Build history of the part. All positions in model axes, mm. A direction names the side the tool comes from. Give positions to 0.01 mm unless a question says otherwise; leave off trailing zeros. Order: outer loops, then holes, each group sorted by start corner. A loop starts at its lowest first (then second) coordinate and runs counter-clockwise, first axis right, second up. Notation, with made-up numbers: (28.25, -21.75) -> (50.25, -21.75) arc R18 ccw to (50.25, 10.25) -> close; hole circle Ø10 at (1, 69.5). An arc over 180 degrees is marked (long way). Use a Markdown table: item, result. Add a question column.
```python
from build123d import *

# Parameters (mm, degrees)
SKETCH1_R                             = 45
BOSS_EXTRUDE1_DEPTH                   = 8
TAP_DRILL_FOR_M2X0_4_TAP1_D           = 1.6
TAP_DRILL_FOR_M2X0_4_TAP1_CSINK_D     = 1.65
TAP_DRILL_FOR_M2X0_4_TAP1_CSINK_ANGLE = 90
SKETCH7_W                             = 6
SKETCH7_H                             = 23.5
CUT_EXTRUDE1_DEPTH                    = 4.1
FILLET1_R                             = 2
BOSS_EXTRUDE2_DEPTH                   = 6
M2_CLEARANCE_HOLE3_D                  = 2.4
SKETCH17_R                            = 1.75
CUT_EXTRUDE2_DEPTH                    = 67.666933473
FILLET1_OF_MIRROR1_R                  = 2


with BuildPart() as part:
    # Sketch1 → Boss-Extrude1 (new body)
    with BuildSketch(Plane(origin=(0, 0, 0), x_dir=(1, 0, 0), z_dir=(0, 1, 0))):
        with Locations(Location((0, 0, 0), (0, 0, 270))):
            Circle(SKETCH1_R)
        Polygon((-15, -36.25), (-15, -4.25), (-20, -4.25), (-20, -5.75), (-26, -5.75), (-26, -4.25), (-34, -4.25), (-34, -11), (-42, -11), (-42, 11), (-34, 11), (-34, 4.25), (-26, 4.25), (-26, 5.75), (-20, 5.75), (-20, 4.25), (-15, 4.25), (-15, 36.25), (15, 36.25), (15, 4.25), (20, 4.25), (20, 5.75), (26, 5.75), (26, 4.25), (34, 4.25), (34, 11), (42, 11), (42, -11), (34, -11), (34, -4.25), (26, -4.25), (26, -5.75), (20, -5.75), (20, -4.25), (15, -4.25), (15, -36.25), align=None, mode=Mode.SUBTRACT)
    extrude(amount=BOSS_EXTRUDE1_DEPTH)

    # Sketch3 → Revolve1 (revolve)
    with BuildSketch(Plane.XY, mode=Mode.PRIVATE) as revolve1_sk:
        with BuildLine():
            Line((-45, 5.8), (-45, 2.2))
            ThreePointArc((-45, 2.2), (-46.8, 4), (-45, 5.8))
        make_face()
    revolve(revolve1_sk.sketch.rotate(Axis((0, 8.4, 0), (0, -1, 0)), 270), axis=Axis((0, 8.4, 0), (0, -1, 0)))

    # Tap Drill for M2x0.4 Tap1 (through all)
    with Locations(Plane(origin=(0, 8, 0), x_dir=(1, 0, 0), z_dir=(0, 1, 0))):
        with Locations((-19.480791822, 19.480791822), (19.480791822, 19.480791822), (19.480791822, -19.480791822), (-19.480791822, -19.480791822)):
            CounterSinkHole(TAP_DRILL_FOR_M2X0_4_TAP1_D / 2, TAP_DRILL_FOR_M2X0_4_TAP1_CSINK_D / 2, counter_sink_angle=TAP_DRILL_FOR_M2X0_4_TAP1_CSINK_ANGLE)

    # Sketch7 → Cut-Extrude1 (cut)
    with BuildSketch(Plane(origin=(0, 8, 0), x_dir=(1, 0, 0), z_dir=(0, 1, 0))):
        with Locations((-23, 0)):
            Rectangle(SKETCH7_W, SKETCH7_H)
    cut_extrude1 = extrude(amount=-CUT_EXTRUDE1_DEPTH, mode=Mode.SUBTRACT)

    # Fillet1
    fillet1_edges = [part.edges().sort_by_distance(p)[0] for p in [
        (-20, 5.95, -11.75),
        (-26, 5.95, 11.75),
        (-26, 5.95, -11.75),
        (-20, 5.95, 11.75),
    ]]
    fillet(fillet1_edges, radius=FILLET1_R)

    # Sketch8 → Boss-Extrude2 (add)
    with BuildSketch(Plane.ZY.offset(20)):
        with BuildLine():
            Line((-5.499090834, 3.9), (-10.499090834, 3.9))
            ThreePointArc((-10.499090834, 3.9), (0, -6.499567055), (10.499090834, 3.9))
            Line((10.499090834, 3.9), (5.499090834, 3.9))
            ThreePointArc((5.499090834, 3.9), (0, -1.5), (-5.499090834, 3.9))
        make_face()
    boss_extrude2 = extrude(amount=BOSS_EXTRUDE2_DEPTH)

    # M2 Clearance Hole3 (through all)
    with Locations(Plane(origin=(0, 3.9, 0), x_dir=(1, 0, 0), z_dir=(0, 1, 0))):
        with Locations((-23, 8.624545417), (-23, -8.624545417)):
            m2_clearance_hole3 = Hole(M2_CLEARANCE_HOLE3_D / 2)

    # Sketch17 → Cut-Extrude2 (cut, through all)
    with BuildSketch(Plane.XZ):
        with Locations((-23, -8.624545417)):
            Circle(SKETCH17_R)
        with Locations((-23, 8.624545417)):
            Circle(SKETCH17_R)
    cut_extrude2 = extrude(amount=CUT_EXTRUDE2_DEPTH, mode=Mode.SUBTRACT)

    # Mirror1: Cut-Extrude1, Boss-Extrude2, M2 Clearance Hole3, Cut-Extrude2 across plane
    add(cut_extrude1.mirror(Plane(origin=(0, 0, 0), x_dir=(0, 0, 1), z_dir=(1, 0, 0))), mode=Mode.SUBTRACT)
    add(boss_extrude2.mirror(Plane(origin=(0, 0, 0), x_dir=(0, 0, 1), z_dir=(1, 0, 0))))
    add(m2_clearance_hole3.mirror(Plane(origin=(0, 0, 0), x_dir=(0, 0, 1), z_dir=(1, 0, 0))), mode=Mode.SUBTRACT)
    add(cut_extrude2.mirror(Plane(origin=(0, 0, 0), x_dir=(0, 0, 1), z_dir=(1, 0, 0))), mode=Mode.SUBTRACT)

    # Fillet1 of Mirror1
    fillet1_of_mirror1_edges = [part.edges().sort_by_distance(p)[0] for p in [
        (20, 5.95, -11.75),
        (26, 5.95, 11.75),
        (26, 5.95, -11.75),
        (20, 5.95, 11.75),
    ]]
    fillet(fillet1_of_mirror1_edges, radius=FILLET1_OF_MIRROR1_R)


solid = part.part
```
(1) Mould opens along Z. For faces 1 (the face through (-30, 4, -4.25)), 2 (the face through (-19, 8, 9)), 3 (the face through (-17.235, 6.885, 41.569)) say: released by +Z, released by -Z, zero draft, split by the parting line, or undercut.
(2) Wall check: probe 1 along X at (y, z) = (7, -0.5); probe 2 along X at (y, z) = (4.25, -9); probe 3 along X at (y, z) = (-4.25, 6). Give the ranges that are in metal, low to high.
(3) Pin check, flat tips, straight feed: pin 1 Ø7.5 at (y, z) = (-3, 3.5) entering from +X; pin 2 Ø6 at (y, z) = (5, 7) entering from +X; pin 3 Ø2 at (x, z) = (-23, 8.62) entering from -Y; pin 4 Ø1.7 at (y, z) = (6, -7) entering from +X. Stop position of each tip, or through.
(4) Band-saw the part on B-B on z = 0. Give the cut face in (x, y), plus the area to 3 significant figures.
(5) Band-saw the part on A-A on x = 0. Give the cut face in (y, z).
(6) Tool access for faces 4 (the face through (23, 6, -11.75)), 5 (the face through (-17.235, 1.085, 41.569)), 6 (the face through (42, 4, 0)): list every direction of +Z, -Z, +X, -X, +Y, -Y with a clear straight run to the whole face (end or side of a thin tool).
Response:
| question | item | result |
|---|---|---|
| 1 | face 1 | undercut |
| 1 | face 2 | zero draft |
| 1 | face 3 | split by the parting line |
| 2 | probe 1 | x = -45 to -42, 42 to 45 |
| 2 | probe 2 | x = -45.91 to -42, -34 to -26, -20 to -15, 15 to 20, 26 to 34, 42 to 45.91 |
| 2 | probe 3 | x = -26 to -20, 20 to 26 |
| 3 | pin 1 | stops at x = 44.98 |
| 3 | pin 2 | stops at x = 46.61 |
| 3 | pin 3 | passes through |
| 3 | pin 4 | stops at x = 45.86 |
| 4 | outline | (-45, 0) -> (-42, 0) -> (-42, 8) -> (-45, 8) -> (-45, 5.8) arc R1.8 ccw to (-45, 2.2) -> close; (-26, -6.5) -> (-20, -6.5) -> (-20, -1.5) -> (-26, -1.5) -> close; (20, -6.5) -> (26, -6.5) -> (26, -1.5) -> (20, -1.5) -> close; (42, 0) -> (45, 0) -> (45, 2.2) arc R1.8 ccw to (45, 5.8) -> (45, 8) -> (42, 8) -> close |
| 4 | area | 118 mm² |
| 5 | outline | (0, -45) -> (2.2, -45) arc R1.8 ccw to (5.8, -45) -> (8, -45) -> (8, -36.25) -> (0, -36.25) -> close; (0, 36.25) -> (8, 36.25) -> (8, 45) -> (5.8, 45) arc R1.8 ccw to (2.2, 45) -> (0, 45) -> close |
| 6 | face 4 | +Y |
| 6 | face 5 | -Y |
| 6 | face 6 | +Y, -Y |
